Check sheet for the modelled part. Datum: model origin and axes. Units: mm. Face numbers are marked on the shaded views. A direction names the side the tool comes from. Round coordinates to 2 decimals unless told otherwise and drop trailing zeros. Write each loop counter-clockwise with the first axis right and the second up, starting at its lowest first coordinate (ties: lowest second). Pieces come first, ordered by that corner, then holes. Notation, with made-up numbers: M 14.5,-13.5 L 41.5,-13.5 A28 ccw 41.5,11.5 Z; hole C 40,-1 d10. An arc over 180 degrees is marked long. One line per item, written item: value.
from build123d import *

# Parameters (mm, degrees)
SKETCH_1_W      = 180
SKETCH_1_H      = 180
EXTRUDE_1_DEPTH = 15
SKETCH_2_W      = 120
SKETCH_2_H      = 120
EXTRUDE_2_DEPTH = 200
SKETCH_3_W      = 300
SKETCH_3_H      = 300
EXTRUDE_3_DEPTH = 15
CHAMFER_1_SIZE  = 20
CHAMFER_2_SIZE  = 5


with BuildPart() as part:
    # 草图1 → 凸台-拉伸1 (new body)
    with BuildSketch(Plane(origin=(0, 0, 0), x_dir=(1, 0, 0), z_dir=(0, 1, 0))):
        Rectangle(SKETCH_1_W, SKETCH_1_H)
    extrude(amount=EXTRUDE_1_DEPTH)

    # 草图2 → 凸台-拉伸2 (add)
    with BuildSketch(Plane.XZ):
        Rectangle(SKETCH_2_W, SKETCH_2_H)
    extrude(amount=EXTRUDE_2_DEPTH)

    # 草图3 → 凸台-拉伸3 (add)
    with BuildSketch(Plane.XZ.offset(200)):
        Rectangle(SKETCH_3_W, SKETCH_3_H)
    extrude(amount=EXTRUDE_3_DEPTH)

    # 倒角1
    chamfer_1_edges = [part.edges().sort_by_distance(p)[0] for p in [
        (-150, -207.5, 150),
        (-150, -207.5, -150),
        (150, -207.5, -150),
        (150, -207.5, 150),
    ]]
    chamfer(chamfer_1_edges, length=CHAMFER_1_SIZE)

    # 倒角2
    chamfer_2_edges = [part.edges().sort_by_distance(p)[0] for p in [
        (-90, 7.5, -90),
        (90, 7.5, -90),
        (90, 7.5, 90),
        (-90, 7.5, 90),
    ]]
    chamfer(chamfer_2_edges, length=CHAMFER_2_SIZE)


solid = part.part
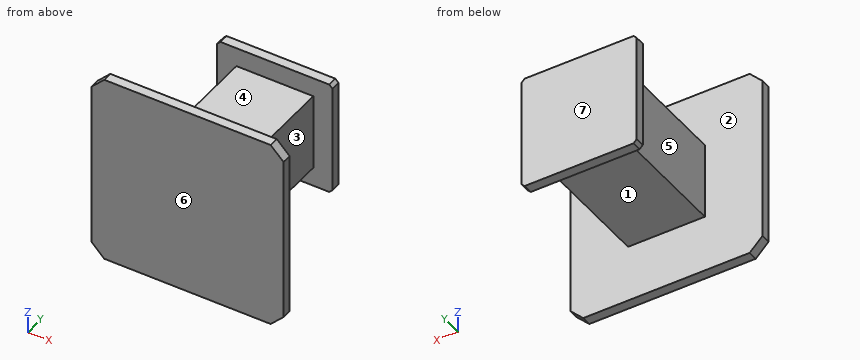
Q1. Scan lines: line 1 (Y direction, x = -36, z = 87.5); line 2 (Y direction, x = 22, z = -125); line 3 (Z direction, x = 23.5, y = -175). Record each from-to range of solid material in increasing order. Write a range as [from, to].
Completed:
line 1: [-215, -200], [0, 15]
line 2: [-215, -200]
line 3: [-60, 60]
Q2. Access from +Z, -Z, +X, -X, +Y, -Y to the whole of each face (thin tool, end or side, straight path). Record for the marked faces 1, 2, 3 and 4.
Completed:
face 1: -Z, +X, -X
face 2: none
face 3: +Z, -Z, +X
face 4: +Z, +X, -X
Q3. Sectioned sample at C-C on z = 11.5. Enter the section's corners in (x, y).
Completed:
outline: M -150,-215 L 150,-215 L 150,-200 L 60,-200 L 60,0 L 90,0 L 90,15 L -90,15 L -90,0 L -60,0 L -60,-200 L -150,-200 Z
Q4. Sectioned sample at A-A on x = 65. Enter the section's corners in (y, z), and give its area (3 significant figures).
Completed:
outline: M -215,-150 L -200,-150 L -200,150 L -215,150 Z; M 0,-90 L 15,-90 L 15,90 L 0,90 Z
area: 7,200 mm^2
Q5. Draft check along Y on the marked faces 5, 6 and 7. Enter one of: pulls with the +Y half, pulls with the -Y half, needs draft (parallel to the pull), parting line crosses it, or undercut.
Completed:
face 5: undercut
face 6: pulls with the -Y half
face 7: pulls with the +Y half
Q6. Sectioned sample at D-D on y = -172. Enter the section's corners in (x, z).
Completed:
outline: M -60,-60 L 60,-60 L 60,60 L -60,60 Z
Q7. Sectioned sample at B-B on x = 18. Enter the section's corners in (y, z), and give its area (3 significant figures).
Completed:
outline: M -215,-150 L -200,-150 L -200,-60 L 0,-60 L 0,-90 L 15,-90 L 15,90 L 0,90 L 0,60 L -200,60 L -200,150 L -215,150 Z
area: 31,200 mm^2
Q8. Depth check by flat-ended pin: P1, Ø8, axis at x = -99.5, z = -89, coming from the +Y side; P2, Ø12, axis at y = 10, z = -41, coming from the -X side; P3, Ø16.5, axis at y = 5, z = 40, coming from the +X side. Enter the tip coordinate at first touch or a pass-through.
Completed:
P1: y = -200
P2: x = -90
P3: x = 90
